Autodesk Inventor part; units mm, degrees
ref_plane "YZ Plane" through (0, 0, 0) normal (1, 0, 0) x (0, 1, 0)
ref_plane "XZ Plane" through (0, 0, 0) normal (0, 1, 0) x (-1, 0, 0)
ref_plane "XY Plane" through (0, 0, 0) normal (0, 0, 1) x (1, 0, 0)
sketch "Sketch1" plane through (0, 0, 0) normal (0, 1, 0) x (-1, 0, 0)
  line L0 (0, 0) -> (-254, 0)
  line L1 (-254, 0) -> (-254, -254)
  line L2 (-254, -254) -> (0, -254)
  line L3 (0, -254) -> (0, 0)
  line L4 (0, -15.875) -> (-10.287, -15.875)
  line L5 (-10.287, -15.875) -> (-10.287, 0)
  line L6 (-243.713, 0) -> (-243.713, -15.875)
  line L7 (-243.713, -15.875) -> (-254, -15.875)
  line L8 (-243.713, -254) -> (-243.713, -238.125)
  line L9 (-243.713, -238.125) -> (-254, -238.125)
  line L10 (-10.287, -254) -> (-10.287, -238.125)
  line L11 (-10.287, -238.125) -> (0, -238.125)
  dimension "d0" = 254
  dimension "d1" = 254
  dimension "d14" = 10.287
  dimension "d15" = 10.287
  dimension "d16" = 15.875
  dimension "d17" = 15.875
extrude "Extrusion1" add sketch "Sketch1" along normal blind 2.286 contours L5 L4 L3 L11 L10 L2 L8 L9 L1 L7 L6 L0
sketch "Sketch2" plane through (0, 2.286, 0) normal (0, 1, 0) x (1, 0, 0)
  line L0 (28.575, 28.575) -> (225.425, 28.575)
  line L1 (225.425, 28.575) -> (225.425, 225.425)
  line L2 (225.425, 225.425) -> (28.575, 225.425)
  line L3 (28.575, 225.425) -> (28.575, 28.575)
  line L4 (0, 15.875) -> (10.287, 15.875)
  line L5 (10.287, 15.875) -> (10.287, 0)
  line L6 (10.287, 0) -> (243.713, 0)
  line L7 (243.713, 0) -> (243.713, 15.875)
  line L8 (243.713, 15.875) -> (254, 15.875)
  line L9 (254, 15.875) -> (254, 238.125)
  line L10 (254, 238.125) -> (243.713, 238.125)
  line L11 (243.713, 238.125) -> (243.713, 254)
  line L12 (243.713, 254) -> (10.287, 254)
  line L13 (10.287, 254) -> (10.287, 238.125)
  line L14 (10.287, 238.125) -> (0, 238.125)
  line L15 (0, 238.125) -> (0, 15.875)
  point P0 (0, 0)
  point P1 (127, 28.575)
  point P2 (127, 0)
  point P3 (28.575, 127)
  point P4 (0, 127)
  dimension "d9" = 196.85
  dimension "d10" = 196.85
extrude "Extrusion2" cut sketch "Sketch2" against normal through all contours L3 L2 L1 L0
sketch "Sketch3" plane through (0, 2.286, 0) normal (0, 1, 0) x (1, 0, 0)
  circle A0 centre (50.8, 9.525) radius 4
  circle A1 centre (203.2, 9.525) radius 4
  circle A2 centre (203.2, 244.475) radius 4.2037
  circle A3 centre (50.8, 244.475) radius 4.2037
  point P0 (0, 0)
hole "Hole1" at (50.8, 2.286, -9.525) at (50.8, 2.286, -244.475) at (203.2, 2.286, -244.475) at (203.2, 2.286, -9.525) direction (0, -1, 0) diameter 15 end through all
chamfer "Chamfer1" distance 3.175 angle 45 1 edges at (0, 1.143, -238.125)
equation "\"d15\" = d14"
equation "\"d17\" = d16"
equation "\"d9\" = d10"
properties part number "Carriage Sheet"
CAD build for the part. Positions are in the model's coordinates, mm. Give positions to 0.01 mm unless a question says otherwise; leave off trailing zeros. Order: outer loops, then holes, each group sorted by start corner. A loop starts at its lowest first (then second) coordinate and runs counter-clockwise, first axis right, second up.
(1) Saw through at C-C, the plane y = 0.85. Give the cut face in (x, z) (3 decimals), then the cut area to 3 significant figures.
(2) Saw through at D-D, the plane x = 155.5. Give the cut face in (y, z) (3 decimals), then the cut area to 3 significant figures.
(3) Flat gauge pins, fed straight in: pin 1 (1.1 mm diameter, centred on x = 7, y = 1.5, fed in from -Z) (3 decimals); pin 2 (0.7 mm diameter, centred on y = 1.5, z = -243.5, fed in from +X); pin 3 (12 mm diameter, centred on x = 50.8, z = -244.475, fed in from +Y). Where does each tip first touch, or does it go through?
(4) Saw through at A-A, the plane x = 50.8. Give the cut face in (y, z) (3 decimals).
(5) Saw through at B-B, the plane z = -124. Give the cut face in (x, y) (3 decimals), then the cut area to 3 significant figures.
(6) Drill centre lines: L1, parallel to Z at x = 50.8, y = 1.35 (3 decimals); L2, parallel to X at y = 1.45, z = -30.5 (3 decimals); L3, parallel to Z at x = 193.5, y = 1.65 (3 decimals). Where is each one in solid material? Low to high.
(7) Mould opens along X. For faces 1 (the flat face through (129, 2.286, -238)), 2 (the cylindrical face through (210.52, 1.13, -11.15)), 3 (the cylindrical face through (53.673, 1.127, -237.547)) say: released by +X, released by -X, zero draft, split by the parting line, or undercut.
Results found:
1. outline: (0, -234.95) - (3.175, -238.125) - (10.287, -238.125) - (10.287, -254) - (243.713, -254) - (243.713, -238.125) - (254, -238.125) - (254, -15.875) - (243.713, -15.875) - (243.713, 0) - (10.287, 0) - (10.287, -15.875) - (0, -15.875) - close; hole (28.575, -225.425) - (225.425, -225.425) - (225.425, -28.575) - (28.575, -28.575) - close; hole circle Ø15 at (50.8, -244.475); hole circle Ø15 at (50.8, -9.525); hole circle Ø15 at (203.2, -244.475); hole circle Ø15 at (203.2, -9.525)
1. area: 24,400 mm2
2. outline: (0, -254) - (2.286, -254) - (2.286, -225.425) - (0, -225.425) - close; (0, -28.575) - (2.286, -28.575) - (2.286, 0) - (0, 0) - close
2. area: 131 mm2
3. pin 1: stops at z = -238.125
3. pin 2: stops at x = 243.71
3. pin 3: passes through
4. outline: (0, -254) - (2.286, -254) - (2.286, -251.975) - (0, -251.975) - close; (0, -236.975) - (2.286, -236.975) - (2.286, -225.425) - (0, -225.425) - close; (0, -28.575) - (2.286, -28.575) - (2.286, -17.025) - (0, -17.025) - close; (0, -2.025) - (2.286, -2.025) - (2.286, 0) - (0, 0) - close
5. outline: (0, 0) - (28.575, 0) - (28.575, 2.286) - (0, 2.286) - close; (225.425, 0) - (254, 0) - (254, 2.286) - (225.425, 2.286) - close
5. area: 131 mm2
6. L1: z = -254 to -251.975, -236.975 to -225.425, -28.575 to -17.025, -2.025 to 0
6. L2: x = 0 to 28.575, 225.425 to 254
6. L3: z = -254 to -225.425, -28.575 to 0
7. face 1: zero draft
7. face 2: undercut
7. face 3: undercut
